Answer from the drawing. Dimensions are ordinates in mm from the lowest x, y and z of the part. Round coordinates to 2 decimals unless told otherwise and drop trailing zeros. Loops run counter-clockwise (first coordinate to the right, second up) from the corner with the lowest first, then second, coordinate; pieces in that order, holes last. Notation, with made-up numbers: M 7,-23 L 62,-23 A11 cw 62,-7 Z; hole C 56.25,41 d2. An arc over 180 degrees is marked long. Answer as CSV lines item,"result".
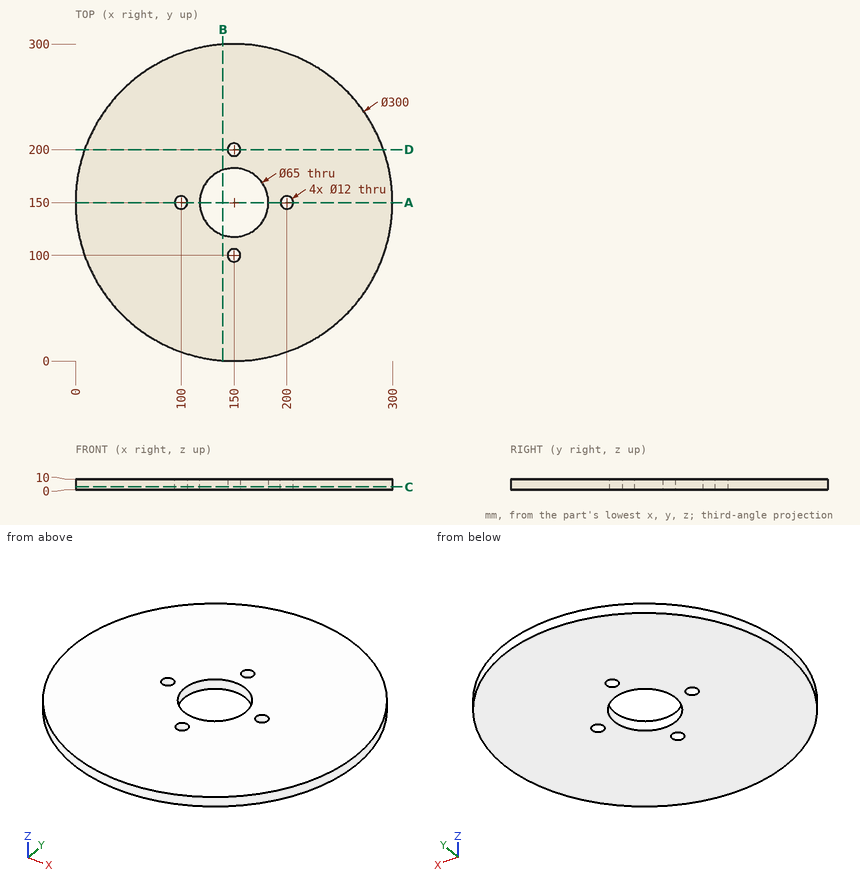
1) Find section C-C, the plane z = 2.5. Give the vertices of the cut face in (x, y).
Evaluation:
outline,"C 150,150 d300; hole C 100,150 d12; hole C 150,150 d65; hole C 150,100 d12; hole C 150,200 d12; hole C 200,150 d12"
2) Find section D-D, the plane y = 200. Give the vertices of the cut face in (x, z), then the cut area to 3 significant figures.
Evaluation:
outline,"M 8.58,0 L 144,0 L 144,10 L 8.58,10 Z; M 156,0 L 291.42,0 L 291.42,10 L 156,10 Z"
area,"2,710 mm^2"
3) Straight lines are drawn through the part: line 1 (Y direction, x = 150, z = 2.5); line 2 (Y direction, x = 94.5, z = 2.5); line 3 (Y direction, x = 170, z = 3.5). For each, find the intervals that lie inside material, in ascending order.
Evaluation:
line 1,"y = 0 to 94, 106 to 117.5, 182.5 to 194, 206 to 300"
line 2,"y = 10.65 to 147.6, 152.4 to 289.35"
line 3,"y = 1.34 to 124.38, 175.62 to 298.66"
4) Each of these flat-tipped pins is pushed along its axis until it touches: P1, Ø4, axis at y = 34, z = 2.5, coming from the +X side; P2, Ø9.5, axis at x = 100, y = 150, coming from the +Z side; P3, Ø6, axis at y = 218, z = 3.5, coming from the +X side; P4, Ø1, axis at x = 124, z = 2, coming from the +Y side. Where does it stop, or does it pass through?
Evaluation:
P1,"stops at x = 247.49"
P2,"passes through"
P3,"stops at x = 285.19"
P4,"stops at y = 297.82"
5) Find section B-B, the plane x = 139.5. Give the vertices of the cut face in (y, z).
Evaluation:
outline,"M 0.37,0 L 119.24,0 L 119.24,10 L 0.37,10 Z; M 180.76,0 L 299.63,0 L 299.63,10 L 180.76,10 Z"
6) Find section A-A, the plane y = 150. Give the vertices of the cut face in (x, z).
Evaluation:
outline,"M 0,0 L 94,0 L 94,10 L 0,10 Z; M 106,0 L 117.5,0 L 117.5,10 L 106,10 Z; M 182.5,0 L 194,0 L 194,10 L 182.5,10 Z; M 206,0 L 300,0 L 300,10 L 206,10 Z"
